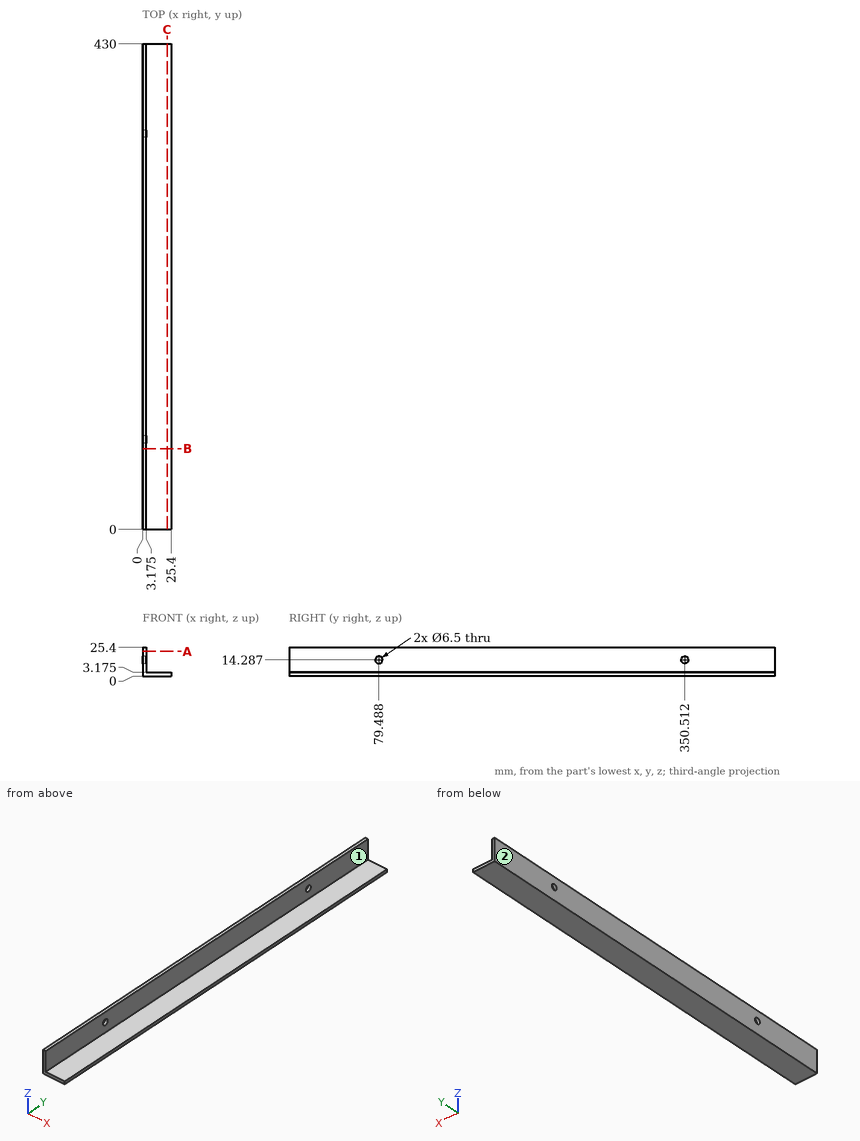
Could you check a few things on this drawing? It's one solid part, dimensions in mm from its lowest x, y, z. A direction names the side the tool comes from. Coordinates: 2 decimals unless noted, no trailing zeros. Order: outer loops, then holes, each group sorted by start corner. A loop starts at its lowest first (then second) coordinate and runs counter-clockwise, first axis right, second up. Notation, with made-up numbers: (83, 1) -> (110, 1) arc R25 cw to (110, 17) -> close; hole circle Ø11 at (-37, -4). An arc over 180 degrees is marked (long way). One line per item, written item: value. Start each with the question number.
1) Imagine slicing it at B-B on y = 71.5. List the corners of the cut face in (x, z) for me (1 decimal).
2) If I drill on L1, parallel to Z at x = 13.75, y = 249 (1 decimal), over which ranges is the centre line in solid material (lowest first)? Write a range as [from, to].
3) Imagine slicing it at C-C on x = 21.75. List the corners of the cut face in (y, z) for me (1 decimal).
4) I'm going to push flat-ended pins straight in: pin 1 (1.5 mm diameter, centred on y = 191.5, z = 8.5, fed in from -X); pin 2 (2 mm diameter, centred on y = 351.5, z = 17, fed in from +X) (1 decimal); pin 3 (1.5 mm diameter, centred on x = 7.5, y = 264, fed in from +Z) (1 decimal). Where does each tip first touch, or does it pass through?
5) Which directions (+Z, -Z, +X, -X, +Y, -Y) give clear straight access to the entire face, cutting with the end or side of a thin tool? Please do the marked faces 1 and 2.
6) Imagine slicing it at A-A on z = 21.75. List the corners of the cut face in (x, y) for me (1 decimal).
Answer list:
1. outline: (0, 0) -> (25.4, 0) -> (25.4, 3.2) -> (3.2, 3.2) -> (3.2, 25.4) -> (0, 25.4) -> close
2. L1: z = [0, 3.2]
3. outline: (0, 0) -> (430, 0) -> (430, 3.2) -> (0, 3.2) -> close
4. pin 1: stops at x = 0
4. pin 2: stops at x = 3.2
4. pin 3: stops at z = 3.2
5. face 1: +Z, +X, +Y, -Y
5. face 2: +Z, -Z, -X, +Y, -Y
6. outline: (0, 0) -> (3.2, 0) -> (3.2, 430) -> (0, 430) -> close
